Read the model definition and answer for the solid it produces. Units are mm, in the model's axes. Face numbers are marked on the shaded views. A direction names the side the tool comes from. Give positions to 0.01 mm unless a question says otherwise; leave off trailing zeros. Order: outer loops, then holes, each group sorted by start corner. A loop starts at its lowest first (then second) coordinate and runs counter-clockwise, first axis right, second up.
Item 1: A cutting plane is placed at C-C (z = -37). Write down the section's boundary in (x, y).
Item 2: A cutting plane is placed at B-B (x = 81). Write down the section's boundary in (y, z), plus the area to 3 significant figures.
Item 3: A cutting plane is placed at A-A (y = 0). Write down the section's boundary in (x, z), plus the area to 3 significant figures.
Item 4: Find the intervals of material crossed by line 1 along Y through (x, z) = (45.5, -6.5); line 2 along X through (y, z) = (-19, -25.5); line 3 along Y through (x, z) = (-10, 6), in increasing order.
Item 5: Given pin 1 Ø4 at (y, z) = (53.5, -21.5) entering from -X; pin 2 Ø2 at (x, z) = (-23.5, -24) entering from +Y; pin 3 Ø22.5 at (x, z) = (-81, 0.5) entering from +Y, each flat-ended and moving along its own axis, determine where each tip first touches the part or whether it passes through.
Item 6: A cutting plane is placed at D-D (x = -153). Write down the section's boundary in (y, z).
Item 7: The mould has two halves that part along Z. Classify the marked faces 6, 7 and 8: +Z half, -Z half, draft (parallel to the pull), parting line (faces both ways), or undercut.
Item 8: Which of the six approach directions +Z, -Z, +X, -X, +Y, -Y give full straight-line access (tool end or side, diameter ignored) to the marked faces 1, 2, 3, 4 and 5?
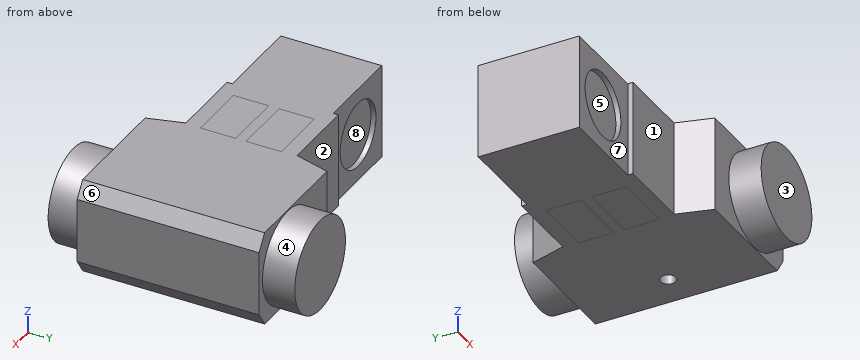
Autodesk Inventor part; units mm, degrees
ref_plane "Work Plane2" through (300, 100, 0) normal (-0.9889364, -0.1483405, 0) x (0.1483405, -0.9889364, 0)
ref_plane "YZ Plane" through (0, 0, 0) normal (1, 0, 0) x (0, 1, 0)
ref_plane "XZ Plane" through (0, 0, 0) normal (0, 1, 0) x (-1, 0, 0)
sketch "Sketch1" plane through (0, 0, 0) normal (0, 0, 1) x (1, 0, 0)
  line L0 (-100, 0) -> (100, 0) construction
  line L1 (-100, 55) -> (-100, -55)
  circle A0 centre (-57.5, 47.5) radius 2.25
  line L2 (100, -70) -> (100, 70) construction
  line L3 (-92, 0) -> (-92, 47.5) construction
  line L4 (-92, 0) -> (-92, -47.5) construction
  circle A1 centre (-92.5, 47.5) radius 2.25
  circle A2 centre (-92.5, 47.5) radius 1.25
  circle A3 centre (-57.5, 47.5) radius 1.25
  line L5 (-100, 55) -> (-33.1573, 55)
  line L6 (-33.1573, 55) -> (-23.1573, 90)
  line L7 (-23.1573, 90) -> (100, 90)
  line L8 (100, 90) -> (100, 0)
  line L9 (100, -90) -> (100, 0)
  line L10 (-23.1573, -90) -> (100, -90)
  line L11 (-33.1573, -55) -> (-23.1573, -90)
  line L12 (-100, -55) -> (-33.1573, -55)
  line L13 (85, 75) -> (-11.8427, 75)
  line L14 (-11.8427, 75) -> (-21.8427, 40)
  line L15 (-21.8427, 40) -> (-92, 40)
  line L16 (-92, -40) -> (-21.8427, -40)
  line L17 (-21.8427, -40) -> (-11.8427, -75)
  line L18 (-11.8427, -75) -> (85, -75)
  line L19 (92.5, 82.5) -> (-17.5, 82.5) construction
  line L20 (-17.5, 82.5) -> (-27.5, 47.5) construction
  line L21 (-27.5, 47.5) -> (-92.5, 47.5) construction
  line L22 (-92.5, 47.5) -> (-92.5, -47.5) construction
  line L23 (-92.5, -47.5) -> (-27.5, -47.5) construction
  line L24 (-27.5, -47.5) -> (-17.5, -82.5) construction
  line L25 (-17.5, -82.5) -> (92.5, -82.5) construction
  line L26 (92.5, -82.5) -> (92.5, 0) construction
  line L27 (92.5, 0) -> (92.5, 82.5) construction
  line L28 (85, 75) -> (85, -75)
  line L29 (-100, 55) -> (-108, 55)
  line L30 (-108, 55) -> (-108, -55)
  line L31 (-108, -55) -> (-100, -55)
  line L32 (-100, -55) -> (-100, 55)
  line L33 (100, 0) -> (-108, 0)
  circle A4 centre (20, 82.5) radius 1.25
  circle A5 centre (20, 82.5) radius 2.25
  circle A6 centre (80, 82.5) radius 1.25
  circle A7 centre (80, 82.5) radius 2.25
  line L34 (50, 90) -> (50, 75) construction
  circle A8 centre (-22.5, 65) radius 1.25
  circle A9 centre (-22.5, 65) radius 2.25
  line L35 (-92, 40) -> (-92, -40)
  circle A10 centre (-96, 0) radius 2.25
  circle A11 centre (-96, 0) radius 1.25
  circle A12 centre (-104, 30) radius 2.25
  circle A13 centre (-104, 30) radius 1.25
  circle A14 centre (-104, -30) radius 2.25
  circle A15 centre (-104, -30) radius 1.25
  line L36 (-104, 55) -> (-104, -55) construction
  line L37 (-32, 40) -> (-32, 5)
  line L38 (-32, 5) -> (-92, 5)
  line L39 (77, 0) -> (77, -50)
  line L40 (77, -50) -> (-3, -50)
  line L41 (-3, -50) -> (-3, 0)
  line L42 (77, -40) -> (67, -40)
  line L43 (67, -40) -> (67, -50)
  line L44 (27, -50) -> (27, -40)
  line L45 (27, -40) -> (17, -40)
  line L46 (17, -40) -> (17, -50)
  circle A16 centre (57, 0) radius 7.5
  point P0 (0, 0)
  point P1 (0, 0)
  point P2 (77, 0)
  point P3 (-3, 0)
  dimension "d0" = 110
  dimension "d1" = 8
  dimension "d2" = 200
  dimension "d15" = 15
  dimension "d17" = 7.5
  dimension "d18" = 4.5
  dimension "d19" = 2.5
  dimension "d20" = 35
  dimension "d21" = 180
  dimension "d22" = 15
  dimension "d24" = 8
  dimension "d28" = 20
  dimension "d29" = 50
  dimension "d30" = 35
  dimension "d40" = 30
  dimension "d41" = 4
  dimension "d110" = 35
  dimension "d111" = 60
  dimension "d114" = 10
  dimension "d115" = 8
  dimension "d132" = 50
  dimension "d133" = 80
  dimension "d135" = 15
  dimension "d138" = 20
  dimension "d139" = 29
  dimension "d140" = 40
  dimension "d141" = 10
  dimension "d155" = 80
sketch "Sketch6" plane through (0, 0, 0) normal (0, 0, 1) x (1, 0, 0)
  line L0 (0, -140) -> (0, 140) construction
  line L1 (60, 0) -> (340, 0) construction
  line L2 (100, -70) -> (100, 70) construction
  line L3 (300, -100) -> (100, -70)
  line L4 (300, 100) -> (100, 70)
  dimension "d146" = 300
  dimension "d147" = 100
ref_plane "Work Plane2" through (300, 100, 0) normal (-0.9889364, -0.1483405, 0) x (0.1483405, -0.9889364, 0)
sketch "Sketch7" plane through (300, 100, 0) normal (-0.9889364, -0.1483405, 0) x (0.1483405, -0.9889364, 0)
  circle A0 centre (0, 0) radius 2.5
  dimension "d150" = 5
extrude "Extrusion1" add sketch "Sketch1" along normal mid plane 94 contours L5 L6 L7 L8 L33 L28 L13 L14 L15 L35 A10 L1 | L1 L33 L30 L29 | L33 A10 L35 L16 L17 L18 L28 L9 L10 L11 L12 L1 | L1 L31 L30 L33 | A10 L33 A11 | L33 A11 A10 | A11 L33 | L33 A11 | L35 L38 L37 L15 L14 L13 L28 L33 A16 | L33 L41 L40 L39 L28 L18 L17 L16 L35 | L33 A16 L39 L42 L43 L40 L44 L45 L46 L41 | L35 L15 L37 L38 | A16 L33 | L33 A16 | L46 L45 L44 L40 | L39 L40 L43 L42 | A0 | A1 | A2 | A3 | A4 | A5 | A6 | A7 | A8 | A9 | A12 | A13 | A14 | A15
extrude "Extrusion2" cut sketch "Sketch1" along normal mid plane 59 contours L35 L38 L37 L15 L14 L13 L28 L33 A16 | L33 L41 L40 L39 L28 L18 L17 L16 L35 | L33 A16 L39 L42 L43 L40 L44 L45 L46 L41 | L35 L15 L37 L38 | A16 L33 | L33 A16 | L46 L45 L44 L40 | L39 L40 L43 L42
sketch "Sketch2" plane through (-108, -55, 47) normal (-1, 0, 0) x (0, 0, 1)
  line L0 (0, -35) -> (0, 145)
  line L1 (-94, 5) -> (0, 5)
  line L2 (0, 5) -> (0, 105)
  line L3 (0, 105) -> (-94, 105)
  line L4 (-94, 105) -> (-94, 5)
  line L5 (-94, 5) -> (0, 105) construction
  line L6 (0, 5) -> (-94, 105) construction
  line L7 (-94, 32) -> (0, 32)
  line L8 (0, 32) -> (0, 78)
  line L9 (0, 78) -> (-94, 78)
  line L10 (-94, 78) -> (-94, 32)
  line L11 (-94, 32) -> (0, 78) construction
  line L12 (0, 32) -> (-94, 78) construction
  point P0 (-47, 55)
  dimension "d52" = 100
  dimension "d55" = 46
extrude "Extrusion3" add sketch "Sketch2" along normal blind 88
extrude "Extrusion4" [suppressed]
sketch "Sketch3" plane through (0, 0, 0) normal (0, 1, 0) x (-1, 0, 0)
  circle A0 centre (153, 0) radius 32.5
  line L0 (108, -47) -> (108, 47)
  line L1 (108, -47) -> (108, 47)
  line L2 (108, -47) -> (108, 47) construction
  line L3 (108, 0) -> (245.8238, 0) construction
  circle A1 centre (153, 0) radius 40
  line L4 (183.942, 9.942) -> (196, 22)
  line L5 (196, 22) -> (196, -22)
  line L6 (196, -22) -> (183.942, -9.942)
  line L7 (196, 47) -> (196, -47)
  line L8 (204, 47) -> (224, 20)
  line L9 (224, 20) -> (224, 47)
  line L10 (224, 47) -> (204, 47)
  line L11 (196, -47) -> (224, -47)
  line L12 (204, -47) -> (224, -20)
  line L13 (224, -20) -> (224, -47)
  line L14 (-100, 47) -> (23.1573, 47)
  line L15 (-100, 47) -> (-100, 32)
  line L16 (-100, 32) -> (-90, 47)
  line L17 (-100, -47) -> (23.1573, -47)
  line L18 (-100, -47) -> (-100, -32)
  line L19 (-100, -32) -> (-90, -47)
  circle A2 centre (-48, 0) radius 46
  line L20 (-100, -47) -> (-100, 47)
  circle A3 centre (-48, 0) radius 32.5
  line L21 (-4.8723, -16) -> (13.1277, -16)
  line L22 (13.1277, -16) -> (13.1277, 16)
  line L23 (13.1277, 16) -> (-4.8723, 16)
  point P0 (0, 0)
  point P1 (189.7631, 15.7631)
  point P2 (189.7631, -15.7631)
  dimension "d58" = 45
  dimension "d59" = 65
  dimension "d62" = 80
  dimension "d64" = 44
  dimension "d69" = 20
  dimension "d70" = 27
  dimension "d80" = 15
  dimension "d81" = 10
  dimension "d87" = 52
  dimension "d88" = 92
  dimension "d116" = 65
  dimension "d121" = 32
  dimension "d122" = 18
  dimension "d134" = 8
  dimension "d143" = 48
extrude "Extrusion15" cut sketch "Sketch3" along normal through all both and the other way through all contours L10 L9 L8 | L12 L13 L11 | L14 L16 L15 | L18 L19 L17
extrude "Extrusion16" add sketch "Sketch1" along normal through all both and the other way through all contours L35 L15 L37 L38
extrude "Extrusion14" add sketch "Sketch3" against normal blind 32 from surface at -90 contours A2 | A3
extrude "Extrusion17" [suppressed]
extrude "Extrusion18" cut sketch "Sketch3" along normal blind 5 from surface at -50 contours A0
extrude "Extrusion21" cut sketch "Sketch1" along normal up to surface (17.5 mm away) from surface at -47 contours A16 L33 | L33 A16
extrude "Extrusion22" add sketch "Sketch1" along normal blind 30 from surface at -29.5 contours L33 A16 L39 L42 L43 L40 L44 L45 L46 L41 | L33 A16 | L46 L45 L44 L40 | L39 L40 L43 L42 picked at (58.4928, -2.6557)
extrude "Extrusion24" [suppressed]
mirror "Mirror2" about plane through (0, 0, 0) normal (0, 1, 0) of "Extrusion14", "Extrusion16", "Extrusion18", "Extrusion22"
equation "\"d17\" = 0.5 * d15"
equation "\"d21\" = d47"
equation "\"d45\" = 124"
equation "\"d46\" = 12"
equation "\"d47\" = 180"
Response values:
1. outline: (-196, -50) - (-108, -50) - (-108, -55) - (-33.16, -55) - (-23.16, -90) - (20.67, -90) - (20.67, -122) - (75.33, -122) - (75.33, -90) - (96.67, -90) - (96.67, 90) - (75.33, 90) - (75.33, 122) - (20.67, 122) - (20.67, 90) - (-23.16, 90) - (-33.16, 55) - (-108, 55) - (-108, 50) - (-196, 50) - close; hole circle Ø15 at (57, 0)
2. outline: (-122, -32.05) - (-90, -32.05) - (-90, -47) - (90, -47) - (90, -32.05) - (122, -32.05) - (122, 32.05) - (90, 32.05) - (90, 47) - (-90, 47) - (-90, 32.05) - (-122, 32.05) - close; hole (-75, -29.5) - (75, -29.5) - (75, 29.5) - (-75, 29.5) - close
2. area: 12,200 mm2
3. outline: (-196, -47) - (49.5, -47) - (49.5, -29.5) - (64.5, -29.5) - (64.5, -47) - (90, -47) - (100, -32) - (100, 32) - (90, 47) - (-196, 47) - close; hole (-92, -29.5) - (-3, -29.5) - (-3, 0.5) - (77, 0.5) - (77, -29.5) - (85, -29.5) - (85, 29.5) - (-92, 29.5) - close
3. area: 19,400 mm2
4. line 1: y = -122 to -75, -50 to 50, 75 to 122
4. line 2: x = -196 to -32, -3 to 77, 85 to 100
4. line 3: y = -90 to -75, 75 to 90
5. pin 1: stops at x = -108
5. pin 2: stops at y = 90
5. pin 3: stops at y = 55
6. outline: (-50, -47) - (50, -47) - (50, -32.5) - (45, -32.5) - (45, 32.5) - (50, 32.5) - (50, 47) - (-50, 47) - (-50, 32.5) - (-45, 32.5) - (-45, -32.5) - (-50, -32.5) - close
7. face 6: +Z half
7. face 7: draft
7. face 8: undercut
8. face 1: +Z, -Z, -X, -Y
8. face 2: +Z, -Z, -X, +Y
8. face 3: +Z, -Z, +X, -X, -Y
8. face 4: +Y
8. face 5: -Y
